from build123d import *

# Parameters (mm, degrees)
F0_W     = 107.1716099977
F0_H     = 6.6367755644
F1_DEPTH = 254


# Not quite as in the source:
# - ends of sketch curves that miss each other by under 0.0002 mm in the source are joined


with BuildPart() as f1:
    # F0 (on Front) → F1 (new body)
    with BuildSketch(Plane.XZ):
        with BuildLine():
            Line((-53.5858049989, -3.3183877822), (-53.5858049989, 3.3183877822))
            add(Edge.make_bspline(
                [(-53.5858049989, 3.3183877822), (-60.7905189574, 3.7842082585), (-74.5629530695, 4.6746644037), (-86.6963968754, 19.2661575582), (-87.1229924092, 29.8680118762), (-87.2426380733, 34.9518884332)],
                knots=[0, 0, 0, 0, 0.3582791422, 0.6848815801, 0.984054993, 0.984054993, 0.984054993, 0.984054993], degree=3))
            ThreePointArc((-87.2426380733, 34.9518884332), (-87.8230310318, 35.1768908631), (-88.0742459033, 35.7464285425))
            Line((-88.0742459033, 35.7464285425), (-93.6096602081, 35.6210684855))
            Line((-93.6096602081, 35.6210684855), (-108.3679497242, 35.286838758))
            Line((-108.3679497242, 35.286838758), (-108.3679497242, -3.3183877822))
            Line((-108.3679497242, -3.3183877822), (-53.5858049989, -3.3183877822))
        make_face()
        with BuildLine():
            add(Edge.make_bspline(
                [(53.5858049989, 3.3183877822), (60.7905189574, 3.7842082585), (74.5629530695, 4.6746644037), (86.6963968754, 19.2661575582), (87.1229924092, 29.8680118762), (87.2426380733, 34.9518884332)],
                knots=[0, 0, 0, 0, 0.3582791422, 0.6848815801, 0.984054993, 0.984054993, 0.984054993, 0.984054993], degree=3))
            Line((53.5858049989, 3.3183877822), (53.5858049989, -3.3183877822))
            Line((53.5858049989, -3.3183877822), (108.3679497242, -3.3183877822))
            Line((108.3679497242, -3.3183877822), (108.3679497242, 35.286838758))
            Line((108.3679497242, 35.286838758), (93.6096602081, 35.6210684855))
            Line((93.6096602081, 35.6210684855), (88.0742459033, 35.7464285425))
            ThreePointArc((88.0742459033, 35.7464285425), (87.8230310318, 35.1768908631), (87.2426380733, 34.9518884332))
        make_face()
        Rectangle(F0_W, F0_H)
        with BuildLine():
            add(Edge.make_bspline(
                [(-87.2426380733, 34.9518884332), (-87.2490148129, 35.2228431489), (-87.2551520855, 35.4938413246), (-87.2612893581, 35.7648395002)],
                knots=[0.984054993, 0.984054993, 0.984054993, 0.984054993, 1, 1, 1, 1], degree=3))
            ThreePointArc((-87.2426380733, 34.9518884332), (-86.6797380364, 35.1964774959), (-86.448124364, 35.7648395002))
            ThreePointArc((-86.448124364, 35.7648395002), (-87.270495427, 36.5779523805), (-88.0742459033, 35.7464285425))
            Line((-88.0742459033, 35.7464285425), (-87.2612893581, 35.7648395002))
        make_face()
        with BuildLine():
            ThreePointArc((-88.0742459033, 35.7464285425), (-87.8230310318, 35.1768908631), (-87.2426380733, 34.9518884332))
            add(Edge.make_bspline(
                [(-87.2426380733, 34.9518884332), (-87.2490148129, 35.2228431489), (-87.2551520855, 35.4938413246), (-87.2612893581, 35.7648395002)],
                knots=[0.984054993, 0.984054993, 0.984054993, 0.984054993, 1, 1, 1, 1], degree=3))
            Line((-87.2612893581, 35.7648395002), (-88.0742459033, 35.7464285425))
        make_face()
        with BuildLine():
            add(Edge.make_bspline(
                [(87.2426380733, 34.9518884332), (87.2490148129, 35.2228431489), (87.2551520855, 35.4938413246), (87.2612893581, 35.7648395002)],
                knots=[0.984054993, 0.984054993, 0.984054993, 0.984054993, 1, 1, 1, 1], degree=3))
            ThreePointArc((87.2426380733, 34.9518884332), (87.8230310318, 35.1768908631), (88.0742459033, 35.7464285425))
            Line((88.0742459033, 35.7464285425), (87.2612893581, 35.7648395002))
        make_face()
        with BuildLine():
            ThreePointArc((88.0744543523, 35.7648395002), (86.6929273539, 36.346390822), (87.2426380733, 34.9518884332))
            add(Edge.make_bspline(
                [(87.2426380733, 34.9518884332), (87.2490148129, 35.2228431489), (87.2551520855, 35.4938413246), (87.2612893581, 35.7648395002)],
                knots=[0.984054993, 0.984054993, 0.984054993, 0.984054993, 1, 1, 1, 1], degree=3))
            Line((87.2612893581, 35.7648395002), (88.0742459033, 35.7464285425))
            ThreePointArc((88.0742459033, 35.7464285425), (88.0744022384, 35.7556334313), (88.0744543523, 35.7648395002))
        make_face()
    extrude(amount=F1_DEPTH)


solid = f1.part
Input: part model. Units: mm. Frame: model coordinates. Give positions to 0.01 mm unless a question says otherwise; leave off trailing zeros. Write each loop counter-clockwise with the first axis right and the second up, starting at its lowest first coordinate (ties: lowest second). Pieces come first, ordered by that corner, then holes.
Q1. First-contact query: P1, Ø12, axis at x = -10.5, z = 10, coming from the -Y side; P2, Ø6, axis at x = 60.5, y = -34, coming from the +Z side. Flat tips, straight axial feed; report the tip coordinate or a pass-through.
Q2. Material intervals for probe 1 along Z at (x, y) = (16.5, -243); probe 2 along X at (y, z) = (-96, 15.5); probe 3 along X at (y, z) = (-14.5, 17), sorted ascending.
Q3. Pull-direction query (X, two-part tool) for faces 1 (the face through (-1, 0, 0)), 2 (the face through (-1, -125, 3.318)), 3 (the face through (108.368, -125, 16)); classes: pulls with the +X half, pulls with the -X half, needs draft (parallel to the pull), parting line crosses it, or undercut.
Q4. Section A-A, the plane x = 10. Output: boundary loops of the cut face in (y, z).
Filled in:
1. P1: passes through
1. P2: stops at z = 4.22
2. probe 1: z = -3.32 to 3.32
2. probe 2: x = -108.37 to -82.7, 82.7 to 108.37
2. probe 3: x = -108.37 to -83.61, 83.61 to 108.37
3. face 1: needs draft
3. face 2: undercut
3. face 3: pulls with the +X half
4. outline: (-254, -3.32) - (0, -3.32) - (0, 3.32) - (-254, 3.32) - close
